Check sheet for the modelled part. Datum: model origin and axes. Units: mm. A direction names the side the tool comes from. Round coordinates to 2 decimals unless told otherwise and drop trailing zeros. Loops run counter-clockwise (first coordinate to the right, second up) from the corner with the lowest first, then second, coordinate; pieces in that order, holes last. Notation, with made-up numbers: (66, -26) - (92, -26) arc R26 cw to (92, 10) - close; hole circle Ø5 at (-14.75, -31.75). An arc over 180 degrees is marked (long way). Put each result on its own line as item: value.
```python
from build123d import *

# Parameters (mm, degrees)
SKETCH_1_R          = 3.4
EXTRUDE_2_DEPTH     = 15
CUT_EXTRUDE_1_DEPTH = 104.680547991
CUT_EXTRUDE_2_DEPTH = 103.721548766
CUT_EXTRUDE_START   = -10
SKETCH_6_R          = 2.5
SKETCH_6_R_2        = 1.6
CUT_EXTRUDE_3_DEPTH = 10
FILLET_1_R          = 5


with BuildPart() as part:
    # 草图1 → 凸台-拉伸2 (new body)
    with BuildSketch(Plane(origin=(0, 0, 0), x_dir=(1, 0, 0), z_dir=(0, 1, 0))):
        with BuildLine():
            ThreePointArc((-7.95357839, 100.709696918), (0.550267992, 75.709696918), (-7.95357839, 50.709696918))
            Line((-7.95357839, 50.709696918), (14.093828565, 50.709696918))
            ThreePointArc((14.093828565, 50.709696918), (19.550267992, 75.709696918), (14.093828565, 100.709696918))
            Line((14.093828565, 100.709696918), (-7.95357839, 100.709696918))
        make_face()
        with Locations(Location((10.36364228, 96.757285698, 0), (0, 0, 270))):
            Circle(SKETCH_1_R, mode=Mode.SUBTRACT)
        with Locations(Location((10.36364228, 54.662108138, 0), (0, 0, 270))):
            Circle(SKETCH_1_R, mode=Mode.SUBTRACT)
    extrude(amount=EXTRUDE_2_DEPTH)

    # 草图2 → 切除-拉伸1 (cut, through all)
    with BuildSketch(Plane(origin=(0, 15, 0), x_dir=(1, 0, 0), z_dir=(0, 1, 0))):
        with BuildLine():
            Line((4.550267992, 88.709696918), (4.550267992, 75.709696918))
            Line((4.550267992, 75.709696918), (19.550267992, 75.709696918))
            ThreePointArc((19.550267992, 75.709696918), (19.192888302, 82.248645039), (18.125006574, 88.709696918))
            Line((18.125006574, 88.709696918), (4.550267992, 88.709696918))
        make_face()
        with BuildLine():
            Line((19.550267992, 75.709696918), (4.550267992, 75.709696918))
            Line((4.550267992, 75.709696918), (4.550267992, 62.709696918))
            Line((4.550267992, 62.709696918), (18.125006574, 62.709696918))
            ThreePointArc((18.125006574, 62.709696918), (19.192888302, 69.170748797), (19.550267992, 75.709696918))
        make_face()
    extrude(amount=-CUT_EXTRUDE_1_DEPTH, mode=Mode.SUBTRACT)

    # 草图4 → 切除-拉伸2 (cut, through all)
    with BuildSketch(Plane(origin=(4.550267992, 0, 0), x_dir=(0, 0, -1), z_dir=(1, 0, 0))):
        with BuildLine():
            ThreePointArc((84.809696918, 7.5), (83.209696918, 9.1), (81.609696918, 7.5))
            Line((81.609696918, 7.5), (84.809696918, 7.5))
        make_face()
        with BuildLine():
            Line((84.809696918, 7.5), (81.609696918, 7.5))
            ThreePointArc((81.609696918, 7.5), (83.209696918, 5.9), (84.809696918, 7.5))
        make_face()
        with BuildLine():
            ThreePointArc((69.809696918, 7.5), (68.209696918, 9.1), (66.609696918, 7.5))
            Line((66.609696918, 7.5), (69.809696918, 7.5))
        make_face()
        with BuildLine():
            Line((69.809696918, 7.5), (66.609696918, 7.5))
            ThreePointArc((66.609696918, 7.5), (68.209696918, 5.9), (69.809696918, 7.5))
        make_face()
    extrude(amount=-CUT_EXTRUDE_2_DEPTH, mode=Mode.SUBTRACT)

    # 草图6 → 切除-拉伸3 (cut)
    # profile 1 of 2: a face of its own
    with BuildSketch(Plane.ZY.offset(7.95357839).offset(CUT_EXTRUDE_START)):
        with Locations((-83.209696918, 7.5)):
            Circle(SKETCH_6_R)
        with Locations(Location((-83.209696918, 7.5, 0), (0, 0, 180))):
            Circle(SKETCH_6_R_2, mode=Mode.SUBTRACT)
    # profile 2 of 2: a face of its own
    with BuildSketch(Plane.ZY.offset(7.95357839).offset(CUT_EXTRUDE_START)):
        with Locations((-68.209696918, 7.5)):
            Circle(SKETCH_6_R)
        with Locations(Location((-68.209696918, 7.5, 0), (0, 0, 180))):
            Circle(SKETCH_6_R_2, mode=Mode.SUBTRACT)
    extrude(amount=CUT_EXTRUDE_3_DEPTH, mode=Mode.SUBTRACT)

    # 圆角1
    fillet_1_edges = [part.edges().sort_by_distance(p)[0] for p in [
        (18.125006574, 7.5, -88.709696918),
        (18.125006574, 7.5, -62.709696918),
    ]]
    fillet(fillet_1_edges, radius=FILLET_1_R)


solid = part.part
```
Item 1: Go/stop test with flat-tipped pins: pin 1 (4.5 mm diameter, centred on y = 7.5, z = -68.21, fed in from -X); pin 2 (5 mm diameter, centred on y = 2.5, z = -80.5, fed in from +X); pin 3 (1.5 mm diameter, centred on y = 7, z = -64.5, fed in from -X). Record where each tip stops, or that it passes through.
Filled sheet:
pin 1: x = 2.05
pin 2: x = 4.55
pin 3: x = -1.23
Item 2: Section check B-B on y = 7.5. Enter the section's corners in (x, z).
Filled sheet:
outline: (-7.95, -100.71) - (14.09, -100.71) arc R60 ccw to (16.25, -95.35) arc R5 ccw to (11.52, -88.71) - (4.55, -88.71) - (4.55, -84.81) - (2.05, -84.81) - (2.05, -85.71) - (-0.69, -85.71) arc R41 cw to start; (-7.95, -50.71) arc R41 cw to (-0.69, -65.71) - (2.05, -65.71) - (2.05, -66.61) - (4.55, -66.61) - (4.55, -62.71) - (11.52, -62.71) arc R5 ccw to (16.25, -56.07) arc R60 ccw to (14.09, -50.71) - close; (0.24, -80.71) - (2.05, -80.71) - (2.05, -81.61) - (4.55, -81.61) - (4.55, -69.81) - (2.05, -69.81) - (2.05, -70.71) - (0.24, -70.71) arc R41 cw to start; hole circle Ø6.8 at (10.36, -96.76); hole circle Ø6.8 at (10.36, -54.66)
Item 3: Section check C-C on y = 13.5. Enter the section's corners in (x, z).
Filled sheet:
outline: (-7.95, -100.71) - (14.09, -100.71) arc R60 ccw to (16.25, -95.35) arc R5 ccw to (11.52, -88.71) - (4.55, -88.71) - (4.55, -62.71) - (11.52, -62.71) arc R5 ccw to (16.25, -56.07) arc R60 ccw to (14.09, -50.71) - (-7.95, -50.71) arc R41 cw to start; hole circle Ø6.8 at (10.36, -96.76); hole circle Ø6.8 at (10.36, -54.66)
Item 4: Tool access check on faces 4 (the cylindrical face through (3.32, 7.43, -69.81)), 5 (the flat face through (4.55, 8, -76)), 6 (the cylindrical face through (0.999, 7.61, -85.707)). Record the directions out of +Z, -Z, +X, -X, +Y, -Y that give a thin tool (end or side, any length) a straight path to the whole face; none if there is none.
Filled sheet:
face 4: +X, -X
face 5: +X, +Y, -Y
face 6: -X
Item 5: Thickness scan on line 1 (Z direction, x = 3.55, y = 7.5); line 2 (Z direction, x = 0.85, y = 7.5); line 3 (Z direction, x = 8.25, y = 3.25). Record the ranges inside material, lowest first. Write a range as from..to.
Filled sheet:
line 1: -100.71..-84.81, -81.61..-69.81, -66.61..-50.71
line 2: -100.71..-85.71, -80.71..-70.71, -65.71..-50.71
line 3: -100.71..-99.42, -94.09..-88.71, -62.71..-57.33, -52..-50.71
Item 6: Section check A-A on x = 6.25. Enter the section's corners in (y, z), then the cut area to 3 significant figures.
Filled sheet:
outline: (0, -100.71) - (15, -100.71) - (15, -88.71) - (0, -88.71) - close; (0, -62.71) - (15, -62.71) - (15, -50.71) - (0, -50.71) - close
area: 360 mm²
Item 7: Release check for a two-part mould opening along Z. For faces 1 (the cylindrical face through (15.22, 7.4, -53.33)), 2 (the flat face through (3, 7, -100.71)), 3 (the flat face through (8, 8, -88.71)) record: +Z half, -Z half, draft (parallel to the pull), parting line (faces both ways), or undercut.
Filled sheet:
face 1: +Z half
face 2: -Z half
face 3: undercut
Item 8: Section check D-D on x = -5.5. Enter the section's corners in (y, z).
Filled sheet:
outline: (0, -100.71) - (15, -100.71) - (15, -97.15) - (0, -97.15) - close; (0, -54.27) - (15, -54.27) - (15, -50.71) - (0, -50.71) - close
